```python
from build123d import *

# Parameters (mm, degrees)
SKETCH1_W           = 254
SKETCH1_H           = 88.9
BOSS_EXTRUDE1_DEPTH = 11.43
FILLET1_R           = 22.86
FILLET2_R           = 22.86
SKETCH2_W           = 11.43
SKETCH2_H           = 43.18
CUT_EXTRUDE1_DEPTH  = 120.65


with BuildPart() as part:
    # Sketch1 → Boss-Extrude1 (new body)
    with BuildSketch(Plane.XY):
        with Locations((127, 44.45)):
            Rectangle(SKETCH1_W, SKETCH1_H)
    extrude(amount=BOSS_EXTRUDE1_DEPTH)

    # Fillet1
    fillet1_edges = [part.edges().sort_by_distance(p)[0] for p in [
        (0, 88.9, 5.715),
    ]]
    fillet(fillet1_edges, radius=FILLET1_R)

    # Fillet2
    fillet2_edges = [part.edges().sort_by_distance(p)[0] for p in [
        (0, 0, 5.715),
    ]]
    fillet(fillet2_edges, radius=FILLET2_R)

    # Sketch2 → Cut-Extrude1 (cut)
    with BuildSketch(Plane.ZY):
        with Locations((5.715, 44.45)):
            Rectangle(SKETCH2_W, SKETCH2_H)
    extrude(amount=-CUT_EXTRUDE1_DEPTH, mode=Mode.SUBTRACT)


solid = part.part
```
Build history of the part. All positions in model axes, mm. A direction names the side the tool comes from. Round coordinates to 2 decimals unless told otherwise and drop trailing zeros. Write each loop counter-clockwise with the first axis right and the second up, starting at its lowest first coordinate (ties: lowest second). Pieces come first, ordered by that corner, then holes.
1) Drill centre lines: probe 1 along Y at (x, z) = (110.5, 4.25); probe 2 along X at (y, z) = (22, 3.25); probe 3 along X at (y, z) = (59.5, 4.5). Where is each one in solid material? Low to high.
2) Band-saw the part on B-B, the plane z = 1.75. List the corners of the cut face in (x, y).
3) Mould opens along Y. For faces 3 (the flat face through (153, 45, 11.43)), 4 (the flat face through (120.65, 45, 6)), 5 (the cylindrical face through (6.519, 6.874, 5.795)), 6 (the flat face through (137, 88.9, 6)) say: +Y half, -Y half, draft (parallel to the pull), parting line (faces both ways), or undercut.
4) Band-saw the part on C-C, the plane y = 27. List the corners of the cut face in (x, z).
5) 3-axis set-ups, long thin cutter, end or side, ignore diameter. For faces 1 (the flat face through (137, 0, 6)), 2 (the flat face through (59, 66.04, 6)): which of +Z, -Z, +X, -X, +Y, -Y reach the whole face in a straight line?
6) Band-saw the part on A-A, the plane x = 64.5. List the corners of the cut face in (y, z).
7) Pin check, flat tip, straight feed: pin 1 (3 mm diameter, centred on x = 179.5, y = 13.5, fed in from -Z). Stop position of the tip, or through.
Ans:
1. probe 1: y = 0 to 22.86, 66.04 to 88.9
1. probe 2: x = 0.02 to 254
1. probe 3: x = 120.65 to 254
2. outline: (0, 22.86) arc R22.86 ccw to (22.86, 0) - (254, 0) - (254, 88.9) - (22.86, 88.9) arc R22.86 ccw to (0, 66.04) - (120.65, 66.04) - (120.65, 22.86) - close
3. face 3: draft
3. face 4: undercut
3. face 5: -Y half
3. face 6: +Y half
4. outline: (120.65, 0) - (254, 0) - (254, 11.43) - (120.65, 11.43) - close
5. face 1: +Z, -Z, +X, -X, -Y
5. face 2: +Z, -Z, -X
6. outline: (0, 0) - (22.86, 0) - (22.86, 11.43) - (0, 11.43) - close; (66.04, 0) - (88.9, 0) - (88.9, 11.43) - (66.04, 11.43) - close
7. pin 1: stops at z = 0
